For this review, take the finished solid that the model builds, in its own axes (mm). A direction names the side the tool comes from. Coordinates: 2 decimals unless noted, no trailing zeros. Order: outer loops, then holes, each group sorted by start corner. A loop starts at its lowest first (then second) coordinate and runs counter-clockwise, first axis right, second up. Notation, with made-up numbers: (47.25, 31.5) -> (92.25, 31.5) arc R20 ccw to (92.25, 35.5) -> close; hole circle Ø11 at (0.5, -24). An arc over 180 degrees is marked (long way). Write item = value, one per line. Start each with the question number.
1) Wall thickness on probe 1 along Y at (x, z) = (295, 297); probe 2 along Y at (x, z) = (152, 296); probe 3 along X at (y, z) = (1419.5, 294): over which ranges is each line inside the solid? List them lowest first. Write a range as [from, to].
2) Consider section B-B on z = 279. State how many separate pieces and enclosed holes the cut face has, and give its area (3 significant figures).
3) Machinability: for faces 5 (the face through (147.714, 1136.858, 279.172)), 6 (the face through (267.982, 1357.535, 274.172)), 7 (the face through (-12.08, 438.12, 279.73)), which of the approach directions +Z, -Z, +X, -X, +Y, -Y give a long, thin tool a straight path to every point of the face, cutting with its end or side? Answer none if there is none.
4) Insertion check: pin 1 Ø8 at (y, z) = (520.5, 280) entering from +X; pin 2 Ø12 at (x, z) = (304, 283) entering from -Y; pin 3 Ø3 at (y, z) = (597, 275.5) entering from -X. Each pin has a flat end and moves straight along its axis. Give the tip position at first contact, or say it passes through.
5) Consider section A-A on y = 1667. Give the boundary of the cut face in (x, z), and give its area (3 significant figures).
6) Draft analysis for pull direction Y (two halves, no side actions). For faces 1 (the face through (125, 913, 254.452)), 2 (the face through (267.92, 38.12, 279.73)), 3 (the face through (152.127, 1577.48, 274.172)), 4 (the face through (387.127, 1577.48, 274.732)), state which applies: +Y half, -Y half, draft (parallel to the pull), parting line (faces both ways), or undercut.
from build123d import *

# Parameters (mm, degrees)
F1_DEPTH  = 1800
F3_DEPTH  = 800
F4_DEPTH  = 600
F5_DEPTH  = 600
F6_DEPTH  = 800
F7_DEPTH  = 600
F8_DEPTH  = 1900
F9_DEPTH  = 1900
F10_DEPTH = 1900
F11_DEPTH = 800


with BuildPart() as f1:
    # F0 (on Front) → F1 (new body)
    with BuildSketch(Plane.XZ):
        Polygon((-134.7514528915, 259.4524627924), (-170.3375428915, 259.4524627924), (-170.3375428915, 254.4524627924), (-130.3375428915, 254.4524627924), (-125.3375428915, 294.4524627924), (104.6624571085, 294.4524627924), (109.6624571085, 254.4524627924), (129.6624571085, 254.4524627924), (129.6624571085, 259.4524627924), (114.0763682012, 259.4524627924), (109.0763682012, 299.4524627924), (-129.7514517988, 299.4524627924), align=None)
        Polygon((-170.3375428915, 299.4524627924), (-170.3375428915, 259.4524627924), (-134.7514528915, 259.4524627924), (-129.7514517988, 299.4524627924), align=None)
        Polygon((150.2485460158, 299.4524627924), (109.0763682012, 299.4524627924), (114.0763682012, 259.4524627924), (129.6624571085, 259.4524627924), (145.2485460158, 259.4524627924), align=None)
        Polygon((389.0763660158, 299.4524627924), (150.2485460158, 299.4524627924), (145.2485460158, 259.4524627924), (129.6624571085, 259.4524627924), (129.6624571085, 254.4524627924), (149.6624571085, 254.4524627924), (154.6624571085, 294.4524627924), (384.6624571085, 294.4524627924), (389.6624571085, 254.4524627924), (429.6624571085, 254.4524627924), (429.6624571085, 259.4524627924), (394.0763671085, 259.4524627924), align=None)
        Polygon((429.6624571085, 299.4524627924), (389.0763660158, 299.4524627924), (394.0763671085, 259.4524627924), (429.6624571085, 259.4524627924), align=None)
    extrude(amount=-F1_DEPTH)

    # F2 (on face) → F3 (cut)
    with BuildSketch(Plane(origin=(-170.3375428915, 0, 0), x_dir=(0, -1, 0), z_dir=(-1, 0, 0))):
        Polygon((-1800, 254.4524627924), (-1760, 254.4524627924), (-1759.375, 259.4524627924), (-1755, 294.4524627924), (-1760.0389110927, 294.4524627924), (-1764.4139110927, 259.4524627924), (-1800, 259.4524627924), align=None)
    extrude(amount=-F3_DEPTH, mode=Mode.SUBTRACT)

    # F2 (on face) → F4 (join)
    with BuildSketch(Plane(origin=(-170.3375428915, 0, 0), x_dir=(0, -1, 0), z_dir=(-1, 0, 0))):
        Polygon((-1760.0389110927, 294.4524627924), (-1759.4139110927, 299.4524627924), (-1800, 299.4524627924), (-1800, 259.4524627924), (-1764.4139110927, 259.4524627924), align=None)
    extrude(amount=-F4_DEPTH)

    # F2 (on face) → F5 (join)
    with BuildSketch(Plane(origin=(-170.3375428915, 0, 0), x_dir=(0, -1, 0), z_dir=(-1, 0, 0))):
        Polygon((-1800, 254.4524627924), (-1760, 254.4524627924), (-1759.375, 259.4524627924), (-1755, 294.4524627924), (-1760.0389110927, 294.4524627924), (-1764.4139110927, 259.4524627924), (-1800, 259.4524627924), align=None)
    extrude(amount=-F5_DEPTH)

    # F2 (on face) → F6 (cut)
    with BuildSketch(Plane(origin=(-170.3375428915, 0, 0), x_dir=(0, -1, 0), z_dir=(-1, 0, 0))):
        Polygon((-1400, 254.4524627924), (-1360, 254.4524627924), (-1355, 294.4524627924), (-1360.0389110927, 294.4524627924), (-1364.4139110927, 259.4524627924), (-1395.5860889073, 259.4524627924), (-1399.9610889073, 294.4524627924), (-1405, 294.4524627924), (-1400.625, 259.4524627924), align=None)
        Polygon((-880.0389110927, 294.4524627924), (-879.4139110927, 299.4524627924), (-900, 299.4524627924), (-900, 259.4524627924), (-884.4139110927, 259.4524627924), align=None)
        Polygon((-920, 254.4524627924), (-900, 254.4524627924), (-900, 259.4524627924), (-915.5860889073, 259.4524627924), (-919.9610889073, 294.4524627924), (-925, 294.4524627924), align=None)
        Polygon((-400.0389110927, 294.4524627924), (-399.4139110927, 299.4524627924), (-440.5860889073, 299.4524627924), (-439.9610889073, 294.4524627924), (-435.5860889073, 259.4524627924), (-404.4139110927, 259.4524627924), align=None)
        Polygon((-35.5860889073, 259.4524627924), (0, 259.4524627924), (0, 299.4524627924), (-40.5860889073, 299.4524627924), (-39.9610889073, 294.4524627924), align=None)
    extrude(amount=-F6_DEPTH, mode=Mode.SUBTRACT)

    # F2 (on face) → F7 (join)
    with BuildSketch(Plane(origin=(-170.3375428915, 0, 0), x_dir=(0, -1, 0), z_dir=(-1, 0, 0))):
        Polygon((-40, 254.4524627924), (0, 254.4524627924), (0, 259.4524627924), (-35.5860889073, 259.4524627924), (-39.9610889073, 294.4524627924), (-45, 294.4524627924), (-40.625, 259.4524627924), align=None)
        Polygon((-440, 254.4524627924), (-400, 254.4524627924), (-399.375, 259.4524627924), (-395, 294.4524627924), (-400.0389110927, 294.4524627924), (-404.4139110927, 259.4524627924), (-435.5860889073, 259.4524627924), (-439.9610889073, 294.4524627924), (-445, 294.4524627924), (-440.625, 259.4524627924), align=None)
        Polygon((-920, 254.4524627924), (-900, 254.4524627924), (-900, 259.4524627924), (-915.5860889073, 259.4524627924), (-919.9610889073, 294.4524627924), (-925, 294.4524627924), align=None)
        Polygon((-915.5860889073, 259.4524627924), (-900, 259.4524627924), (-900, 299.4524627924), (-920.5860889073, 299.4524627924), (-919.9610889073, 294.4524627924), align=None)
        Polygon((-900, 254.4524627924), (-880, 254.4524627924), (-879.375, 259.4524627924), (-875, 294.4524627924), (-880.0389110927, 294.4524627924), (-884.4139110927, 259.4524627924), (-900, 259.4524627924), align=None)
        Polygon((-1400, 254.4524627924), (-1360, 254.4524627924), (-1355, 294.4524627924), (-1360.0389110927, 294.4524627924), (-1364.4139110927, 259.4524627924), (-1395.5860889073, 259.4524627924), (-1399.9610889073, 294.4524627924), (-1405, 294.4524627924), (-1400.625, 259.4524627924), align=None)
        Polygon((-1360.0389110927, 294.4524627924), (-1359.4139110927, 299.4524627924), (-1400.5860889073, 299.4524627924), (-1399.9610889073, 294.4524627924), (-1395.5860889073, 259.4524627924), (-1364.4139110927, 259.4524627924), align=None)
    extrude(amount=-F7_DEPTH)

    # F0 (on Front) → F8 (cut)
    with BuildSketch(Plane.XZ):
        Polygon((-170.3375428915, 299.4524627924), (-170.3375428915, 259.4524627924), (-134.7514528915, 259.4524627924), (-129.7514517988, 299.4524627924), align=None)
    extrude(amount=-F8_DEPTH, mode=Mode.SUBTRACT)

    # F0 (on Front) → F9 (cut)
    with BuildSketch(Plane.XZ):
        Polygon((150.2485460158, 299.4524627924), (109.0763682012, 299.4524627924), (114.0763682012, 259.4524627924), (129.6624571085, 259.4524627924), (145.2485460158, 259.4524627924), align=None)
    extrude(amount=-F9_DEPTH, mode=Mode.SUBTRACT)

    # F0 (on Front) → F10 (cut)
    with BuildSketch(Plane.XZ):
        Polygon((429.6624571085, 299.4524627924), (389.0763660158, 299.4524627924), (394.0763671085, 259.4524627924), (429.6624571085, 259.4524627924), align=None)
    extrude(amount=-F10_DEPTH, mode=Mode.SUBTRACT)

    # F2 (on face) → F11 (cut)
    with BuildSketch(Plane(origin=(-170.3375428915, 0, 0), x_dir=(0, -1, 0), z_dir=(-1, 0, 0))):
        Polygon((-1760.0389110927, 294.4524627924), (-1759.4139110927, 299.4524627924), (-1800, 299.4524627924), (-1800, 259.4524627924), (-1764.4139110927, 259.4524627924), align=None)
        Polygon((-1360.0389110927, 294.4524627924), (-1359.4139110927, 299.4524627924), (-1400.5860889073, 299.4524627924), (-1399.9610889073, 294.4524627924), (-1395.5860889073, 259.4524627924), (-1364.4139110927, 259.4524627924), align=None)
        Polygon((-915.5860889073, 259.4524627924), (-900, 259.4524627924), (-900, 299.4524627924), (-920.5860889073, 299.4524627924), (-919.9610889073, 294.4524627924), align=None)
    extrude(amount=-F11_DEPTH, mode=Mode.SUBTRACT)


solid = f1.part
Answer sheet:
q1.probe_1 = [40.28, 399.72], [440.28, 879.72], [920.28, 1359.72], [1400.28, 1759.72]
q1.probe_2 = [40.15, 399.85], [440.15, 879.85], [920.15, 1359.85], [1400.15, 1759.85]
q1.probe_3 = [-130.43, -125.39], [104.72, 109.76], [149.57, 154.61], [384.72, 389.76]
q2.separate_pieces = 8
q2.enclosed_holes = 8
q2.area = 51,400 mm2
q3.face_5 = +Z, +Y, -Y
q3.face_6 = -Z
q3.face_7 = +Z, +X, -X
q4.pin_1 = 392.01
q4.pin_2 = 37.78
q4.pin_3 = -132.93
q5.outline = (-170.34, 254.45) -> (-130.34, 254.45) -> (-125.34, 294.45) -> (104.66, 294.45) -> (109.66, 254.45) -> (149.66, 254.45) -> (154.66, 294.45) -> (384.66, 294.45) -> (389.66, 254.45) -> (429.66, 254.45) -> (429.66, 259.45) -> (394.08, 259.45) -> (389.08, 299.45) -> (150.25, 299.45) -> (145.25, 259.45) -> (114.08, 259.45) -> (109.08, 299.45) -> (-129.75, 299.45) -> (-134.75, 259.45) -> (-170.34, 259.45) -> close
q5.area = 3,710 mm2
q6.face_1 = draft
q6.face_2 = -Y half
q6.face_3 = undercut
q6.face_4 = undercut
